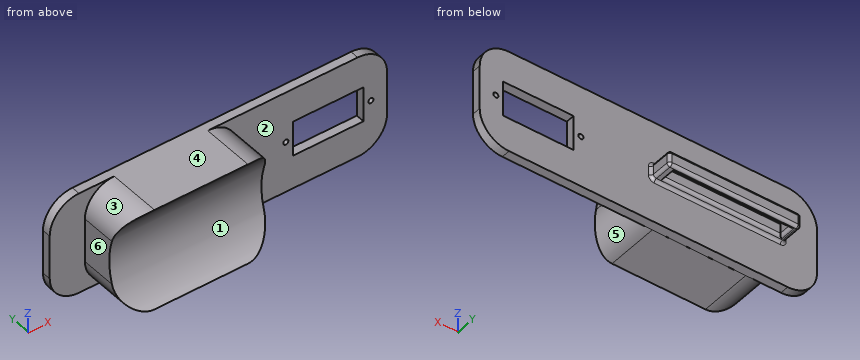
from build123d import *

# Parameters (mm, degrees)
SKETCH1_W           = 115
SKETCH1_H           = 35
BOSS_EXTRUDE1_DEPTH = 3
FILLET1_R           = 10
SKETCH2_W           = 45
SKETCH2_H           = 5
BOSS_EXTRUDE2_DEPTH = 8
SKETCH3_W           = 40
SKETCH3_H           = 4
CUT_EXTRUDE1_DEPTH  = 62.763488753
FILLET2_R           = 1
SKETCH4_W           = 24
SKETCH4_H           = 12
CUT_EXTRUDE2_DEPTH  = 61.634148794
BOSS_EXTRUDE3_DEPTH = 18
FILLET3_R           = 10
FILLET4_R           = 10
SKETCH12_R          = 0.875
CUT_EXTRUDE3_DEPTH  = 64.675135077
CUT_EXTRUDE4_DEPTH  = 58


# Some blends are built 0.0001 mm under size
with BuildPart() as part:
    # Sketch1 → Boss-Extrude1 (new body)
    with BuildSketch(Plane(origin=(0, 0, 0), x_dir=(1, 0, 0), z_dir=(0, 1, 0))):
        Rectangle(SKETCH1_W, SKETCH1_H)
    extrude(amount=BOSS_EXTRUDE1_DEPTH)

    # Fillet1
    fillet1_edges = [part.edges().sort_by_distance(p)[0] for p in [
        (-57.5, 1.5, -17.5),
        (57.5, 1.5, -17.5),
        (57.5, 1.5, 17.5),
        (-57.5, 1.5, 17.5),
    ]]
    fillet(fillet1_edges, radius=FILLET1_R)

    # Sketch2 → Boss-Extrude2 (add)
    with BuildSketch(Plane(origin=(0, 3, 0), x_dir=(1, 0, 0), z_dir=(0, 1, 0))):
        with Locations((-23.5, 0.315525333)):
            Rectangle(SKETCH2_W, SKETCH2_H)
    extrude(amount=BOSS_EXTRUDE2_DEPTH)

    # Sketch3 → Cut-Extrude1 (cut, through all)
    with BuildSketch(Plane.XY.offset(2.184474667)):
        with Locations((-23.5, 7)):
            Rectangle(SKETCH3_W, SKETCH3_H)
    extrude(amount=-CUT_EXTRUDE1_DEPTH, mode=Mode.SUBTRACT)

    # Fillet2
    fillet2_edges = [part.edges().sort_by_distance(p)[0] for p in [
        (-1, 3, -0.315525333),
        (-1, 7, 2.184474667),
        (-23.5, 3, -2.815525333),
        (-1, 7, -2.815525333),
        (-46, 3, -0.315525333),
        (-46, 7, -2.815525333),
        (-23.5, 3, 2.184474667),
        (-46, 7, 2.184474667),
        (-1, 11, -0.315525333),
        (-23.5, 11, -2.815525333),
        (-46, 11, -0.315525333),
        (-23.5, 11, 2.184474667),
        (-43.5, 7, -2.815525333),
        (-23.5, 9, -2.815525333),
        (-23.5, 5, -2.815525333),
        (-43.5, 7, 2.184474667),
        (-23.5, 5, 2.184474667),
        (-3.5, 7, 2.184474667),
        (-23.5, 9, 2.184474667),
    ]]
    fillet(fillet2_edges, radius=FILLET2_R - 0.0001)  # a hair under: the kernel refuses the full size

    # Sketch4 → Cut-Extrude2 (cut, through all)
    with BuildSketch(Plane(origin=(0, 3, 0), x_dir=(1, 0, 0), z_dir=(0, 1, 0))):
        with Locations((37.5, 0)):
            Rectangle(SKETCH4_W, SKETCH4_H)
    extrude(amount=-CUT_EXTRUDE2_DEPTH, mode=Mode.SUBTRACT)

    # Sketch11 → Boss-Extrude3 (add)
    with BuildSketch(Plane(origin=(0, 0, 0), x_dir=(-1, 0, 0), z_dir=(0, -1, 0))):
        Polygon((-6.369569975, 0), (-6.369569975, -17.5), (45.499835489, -17.5), (45.499835489, 17.536176175), (-6.369569975, 17.5), align=None)
    extrude(amount=BOSS_EXTRUDE3_DEPTH)

    # Fillet3
    # the kernel refuses this fillet: 10 mm, written as the material it takes off along each edge
    with BuildSketch(Plane(origin=(-45.499835489, 0, 17.5), x_dir=(1, 0, 0), z_dir=(0, -1, 0))) as fillet3_piece_1:
        with BuildLine():
            CenterArc((FILLET3_R, -FILLET3_R), FILLET3_R, 90, 90)
            Line((0, -FILLET3_R), (0, 0))
            Line((0, 0), (FILLET3_R, 0))
        make_face()
    extrude(amount=43, mode=Mode.SUBTRACT)
    with BuildSketch(Plane(origin=(-45.499835489, 0, -17.536176175), x_dir=(0, 0, 1), z_dir=(0, -1, 0))) as fillet3_piece_2:
        with BuildLine():
            CenterArc((FILLET3_R * 1.00069769048, -FILLET3_R), FILLET3_R, 90, 90.039960778)
            Line((FILLET3_R * 0.000697933699006, -FILLET3_R * 1.0006974471), (0, 0))
            Line((0, 0), (FILLET3_R * 1.00069769048, 0))
        make_face()
    extrude(amount=43.017442262, mode=Mode.SUBTRACT)

    # Fillet4
    # the kernel refuses this fillet: 10 mm, written as the material it takes off along each edge
    with BuildSketch(Plane(origin=(6.369569975, 0, -17.5), x_dir=(0, 0, 1), z_dir=(0, -1, 0))) as fillet4_piece_1:
        with BuildLine():
            CenterArc((FILLET4_R * 0.99930279595, FILLET4_R), FILLET4_R, 180.039960778, 89.960039222)
            Line((-FILLET4_R * 0.000696960833864, FILLET4_R * 0.999302552903), (0, 0))
            Line((0, 0), (FILLET4_R * 0.99930279595, 0))
        make_face()
    extrude(amount=42.982569899, mode=Mode.SUBTRACT)
    with BuildSketch(Plane(origin=(6.369569975, 0, 17.5), x_dir=(0, 0, -1), z_dir=(0, -1, 0))) as fillet4_piece_2:
        with BuildLine():
            CenterArc((FILLET4_R, -FILLET4_R), FILLET4_R, 90, 90)
            Line((0, -FILLET4_R), (0, 0))
            Line((0, 0), (FILLET4_R, 0))
        make_face()
    extrude(amount=43, mode=Mode.SUBTRACT)

    # Sketch12 → Cut-Extrude3 (cut, through all)
    with BuildSketch(Plane(origin=(0, 3, 0), x_dir=(1, 0, 0), z_dir=(0, 1, 0))):
        with Locations(Location((23, 0, 0), (0, 0, 270))):
            Circle(SKETCH12_R)
        with Locations(Location((52, 0, 0), (0, 0, 270))):
            Circle(SKETCH12_R)
    extrude(amount=-CUT_EXTRUDE3_DEPTH, mode=Mode.SUBTRACT)

    # Sketch13 → Cut-Extrude4 (cut)
    with BuildSketch(Plane.ZY.offset(45.499835489)):
        with BuildLine():
            Line((-17.52919927, -18), (17.5, -18))
            ThreePointArc((17.5, -18), (-0.014599635, -10.875312322), (-17.52919927, -18))
        make_face()
    extrude(amount=-CUT_EXTRUDE4_DEPTH, mode=Mode.SUBTRACT)


solid = part.part
Read the model definition and answer for the solid it produces. Units are mm, in the model's axes. Face numbers are marked on the shaded views. A direction names the side the tool comes from. Round coordinates to 2 decimals unless told otherwise and drop trailing zeros. Write each loop counter-clockwise with the first axis right and the second up, starting at its lowest first coordinate (ties: lowest second). Pieces come first, ordered by that corner, then holes.
1. Given pin 1 Ø5 at (x, y) = (6.5, -6) entering from -Z; pin 2 Ø0.9 at (y, z) = (6.5, -0.5) entering from +X; pin 3 Ø0.9 at (x, y) = (-1.5, 2) entering from -Z, each flat-ended and moving along its own axis, determine where each tip first touches the part or whether it passes through.
2. Determine the mould class of the marked faces 1, 2 and 3 for opening direction Z: pulls with the +Z half, pulls with the -Z half, needs draft (parallel to the pull), parting line crosses it, or undercut.
3. The part is cut by section C-C, the plane y = -3.25. Determine the outline of the cut face in (x, z), then the cut area to 3 significant figures.
4. Which of the six approach directions +Z, -Z, +X, -X, +Y, -Y give full straight-line access (tool end or side, diameter ignored) to the marked faces 4, 5 and 6?
5. The part is cut by section D-D, the plane z = 10.5. Determine the outline of the cut face in (x, y), then the cut area to 3 significant figures.
6. Straight lines are drawn through the part: L1, parallel to X at y = 1.45, z = 0 (3 decimals); L2, parallel to X at y = -4.25, z = 2; L3, parallel to Y at x = 10, z = 0.5. For each, find the intervals that lie inside material, in ascending order.
7. The part is cut by section A-A, the plane y = 6. Determine the outline of the cut face in (x, z), then the cut area to 3 significant figures.
8. The part is cut by section B-B, the plane x = 31. Determine the outline of the cut face in (y, z).
Values:
1. pin 1: stops at z = -13.97
1. pin 2: stops at x = -1
1. pin 3: stops at z = -17.5
2. face 1: undercut
2. face 2: needs draft
2. face 3: pulls with the +Z half
3. outline: (-45.5, -7.53) arc R10 ccw to (-35.49, -17.53) - (-3.62, -17.51) arc R10 ccw to (6.37, -7.51) - (6.37, 7.5) arc R10 ccw to (-3.63, 17.5) - (-35.5, 17.5) arc R10 ccw to (-45.5, 7.5) - close
3. area: 1,730 mm2
4. face 4: +Z, +X, -X, +Y, -Y
4. face 5: -Z, +X, -Y
4. face 6: +Z, -Z, -X, -Y
5. outline: (-57.04, 0) - (-45.04, 0) - (-45.04, -13.18) - (5.91, -13.18) - (5.91, 0) - (57.04, 0) - (57.04, 3) - (-57.04, 3) - close
5. area: 1,010 mm2
6. L1: x = -57.5 to 22.125, 23.875 to 25.5, 49.5 to 51.125, 52.875 to 57.5
6. L2: x = -45.5 to 6.37
6. L3: y = 0 to 3
7. outline: (-46, -1.82) arc R1 ccw to (-45, -2.82) - (-44.5, -2.82) arc R1 ccw to (-43.5, -1.82) - (-43.5, 1.18) arc R1 ccw to (-44.5, 2.18) - (-45, 2.18) arc R1 ccw to (-46, 1.18) - close; (-3.5, -2.82) - (-2, -2.82) arc R1 ccw to (-1, -1.82) - (-1, 1.18) arc R1 ccw to (-2, 2.18) - (-2.5, 2.18) arc R1 ccw to (-3.5, 1.18) - close
7. area: 23.5 mm2
8. outline: (0, -17.5) - (3, -17.5) - (3, -6) - (0, -6) - close; (0, 6) - (3, 6) - (3, 17.5) - (0, 17.5) - close
